Verification items for the finished model (mm, model axes). A direction names the side the tool comes from. Round coordinates to 2 decimals unless told otherwise and drop trailing zeros. Order: outer loops, then holes, each group sorted by start corner. A loop starts at its lowest first (then second) coordinate and runs counter-clockwise, first axis right, second up. Notation, with made-up numbers: (-31.5, 15) -> (-2.5, 15) arc R36 ccw to (-2.5, 50) -> close; hole circle Ø2 at (20.25, 71.25). An arc over 180 degrees is marked (long way). Return JSON: item names as keys, results as strings. Group by question number.
Item 1: Draft check along Y on faces 1 (the flat face through (3, 9.5, 7)), 2 (the flat face through (0, 8, 8)), 3 (the flat face through (3, -9.5, 7)), 4 (the flat face through (4, -7.5, 8)). Enter one of: pulls with the +Y half, pulls with the -Y half, needs draft (parallel to the pull), parting line crosses it, or undercut.
Item 2: Sectioned sample at A-A on z = 3.25. Record the cut outline in (x, y), plus the area to 3 significant figures.
Item 3: Sectioned sample at C-C on x = 5. Record the cut outline in (y, z), plus the area to 3 significant figures.
Item 4: Depth check by flat-ended pin: pin 1 Ø6 at (y, z) = (7.5, 11.5) entering from -X; pin 2 Ø2 at (x, z) = (-0.5, 11) entering from +Y; pin 3 Ø2 at (x, z) = (5, 10) entering from +Y; pin 4 Ø4 at (x, y) = (-1.5, -3) entering from +Z. Enter the tip coordinate at first touch or a pass-through.
Item 5: Scan lines: probe 1 along X at (y, z) = (-8, 10); probe 2 along Y at (x, z) = (2, 5.5); probe 3 along Z at (x, y) = (0, 5.75). Record each from-to range of solid material in increasing order. Write a range as from..to.
Item 6: Sectioned sample at D-D on x = -4. Record the cut outline in (y, z).
Item 7: Sectioned sample at B-B on y = 8.25. Record the cut outline in (x, z).
Item 8: Access from +Z, -Z, +X, -X, +Y, -Y to the whole of each face (thin tool, end or side, straight path). Record for faces 5 (the flat face through (0, -9, 8)), 6 (the flat face through (0, 0, 1)), 7 (the cylindrical face through (4.24, -8.51, 10.99)).
```python
from build123d import *

# Parameters (mm, degrees)
EXTRUDE_1_DEPTH     = 2
SKETCH_3_W          = 8
SKETCH_3_H          = 2
EXTRUDE_2_DEPTH     = 12
SKETCH_11_R         = 1.25
CUT_EXTRUDE_3_DEPTH = 25.919871589
CUT_EXTRUDE_4_REACH = 19.27
SKETCH_10_R         = 0.5


with BuildPart() as part:
    # 草图2 → 凸台-拉伸1 (new body)
    with BuildSketch(Plane.XY):
        Polygon((-4.9, -9.5), (8, -9.5), (8, 9.5), (-4.9, 9.5), (-4.9, 5.5), (0, 5.5), (0, -5.5), (-4.9, -5.5), align=None)
    extrude(amount=EXTRUDE_1_DEPTH)

    # 草图3 → 凸台-拉伸2 (add)
    with BuildSketch(Plane.XY.offset(2)):
        with Locations((4, 8.5)):
            Rectangle(SKETCH_3_W, SKETCH_3_H)
        with Locations((4, -8.5)):
            Rectangle(SKETCH_3_W, SKETCH_3_H)
    extrude(amount=EXTRUDE_2_DEPTH)

    # 草图11 → 切除-拉伸3 (cut, through all)
    with BuildSketch(Plane.XZ.offset(9.5)):
        with Locations(Location((5, 10, 0), (0, 0, 270))):
            Circle(SKETCH_11_R)
    extrude(amount=-CUT_EXTRUDE_3_DEPTH, mode=Mode.SUBTRACT)

    # 草图10 → 切除-拉伸4 (cut, up to next)
    with BuildSketch(Plane.XY.offset(2), mode=Mode.PRIVATE) as cut_extrude_4_sk1:
        with Locations((-3, 7.5)):
            Circle(SKETCH_10_R)
    cut_extrude_4_tool1 = extrude(cut_extrude_4_sk1.sketch, amount=-CUT_EXTRUDE_4_REACH, mode=Mode.PRIVATE) & part.part
    # 草图10 → 切除-拉伸4 (cut, up to next)
    with BuildSketch(Plane.XY.offset(2), mode=Mode.PRIVATE) as cut_extrude_4_sk2:
        with Locations((-3, -7.5)):
            Circle(SKETCH_10_R)
    cut_extrude_4_tool2 = extrude(cut_extrude_4_sk2.sketch, amount=-CUT_EXTRUDE_4_REACH, mode=Mode.PRIVATE) & part.part
    add(cut_extrude_4_tool1.solids().sort_by_distance((-3, 7.5, 2))[0], mode=Mode.SUBTRACT)
    add(cut_extrude_4_tool2.solids().sort_by_distance((-3, -7.5, 2))[0], mode=Mode.SUBTRACT)


solid = part.part
```
Recorded:
{
 "1": {"face 1": "pulls with the +Y half", "face 2": "needs draft", "face 3": "pulls with the -Y half", "face 4": "undercut"},
 "2": {"outline": "(0, -9.5) -> (8, -9.5) -> (8, -7.5) -> (0, -7.5) -> close; (0, 7.5) -> (8, 7.5) -> (8, 9.5) -> (0, 9.5) -> close", "area": "32.0 mm²"},
 "3": {"outline": "(-9.5, 0) -> (9.5, 0) -> (9.5, 8.75) -> (7.5, 8.75) -> (7.5, 2) -> (-7.5, 2) -> (-7.5, 8.75) -> (-9.5, 8.75) -> close; (-9.5, 11.25) -> (-7.5, 11.25) -> (-7.5, 14) -> (-9.5, 14) -> close; (7.5, 11.25) -> (9.5, 11.25) -> (9.5, 14) -> (7.5, 14) -> close", "area": "76.0 mm²"},
 "4": {"pin 1": "x = 0", "pin 2": "y = 9.5", "pin 3": "through", "pin 4": "z = 2"},
 "5": {"probe 1": "0..3.75, 6.25..8", "probe 2": "-9.5..-7.5, 7.5..9.5", "probe 3": "0..2"},
 "6": {"outline": "(-9.5, 0) -> (-5.5, 0) -> (-5.5, 2) -> (-9.5, 2) -> close; (5.5, 0) -> (9.5, 0) -> (9.5, 2) -> (5.5, 2) -> close"},
 "7": {"outline": "(-4.9, 0) -> (8, 0) -> (8, 14) -> (0, 14) -> (0, 2) -> (-4.9, 2) -> close; hole circle Ø2.5 at (5, 10)"},
 "8": {"face 5": "+Z, -X, +Y, -Y", "face 6": "+Z, -Z, -X", "face 7": "+Y, -Y"}
}
